The listing builds one solid part. Answer for the finished solid, in the listing's coordinates (mm). Face numbers are marked on the shaded views. A direction names the side the tool comes from. Coordinates: 2 decimals unless noted, no trailing zeros. Order: outer loops, then holes, each group sorted by start corner. A loop starts at its lowest first (then second) coordinate and runs counter-clockwise, first axis right, second up.
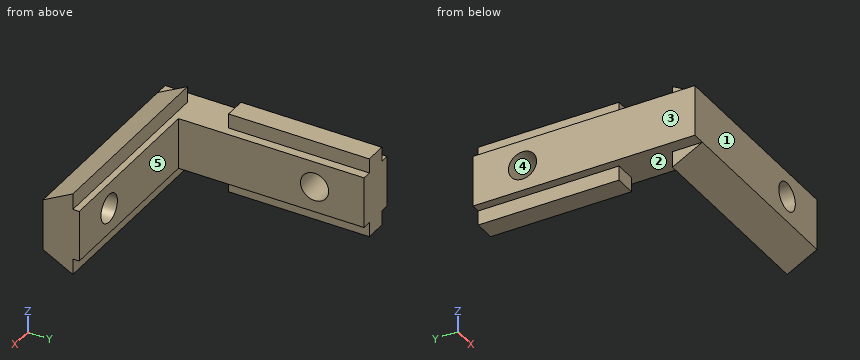
```python
from build123d import *

# Parameters (mm, degrees)
BOSS_EXTRUDE1_DEPTH   = 3
BOSS_EXTRUDE2_DEPTH   = 24
SKETCH3_W             = 1.3
SKETCH3_H             = 10.4
BOSS_EXTRUDE3_DEPTH   = 16.5
M4X0_7_TAPPED_HOLE1_D = 3.3
M4X0_7_TAPPED_HOLE2_D = 3.3
SKETCH9_W             = 3
SKETCH9_H             = 3
CUT_EXTRUDE1_DEPTH    = 38.329478968
MOVE_FACE1_BY         = 0.75
MOVE_FACE2_BY         = 0.4
MOVE_FACE3_BY         = 0.75
MOVE_FACE3_2_BY       = 0.75
MOVE_FACE4_BY         = 0.45
MOVE_FACE4_2_BY       = 0.45
MOVE_FACE5_BY         = 0.5
MOVE_FACE5_2_BY       = 0.5
MOVE_FACE6_BY         = 1
MOVE_FACE8_BY         = 0.25
MOVE_FACE8_2_BY       = 0.25


with BuildPart() as part:
    # Sketch1 → Boss-Extrude1 (new, symmetric)
    with BuildSketch(Plane.XY):
        with BuildLine():
            Line((0, 26), (0, 0))
            Line((0, 0), (25.5, 0))
            Line((25.5, 0), (25.5, 5))
            Line((25.5, 5), (8, 5))
            ThreePointArc((8, 5), (5.878679656, 5.878679656), (5, 8))
            Line((5, 8), (5, 26))
            Line((5, 26), (0, 26))
        make_face()
    extrude(amount=BOSS_EXTRUDE1_DEPTH, both=True)

    # Sketch2 → Boss-Extrude2 (add)
    with BuildSketch(Plane(origin=(25.5, 0, 0), x_dir=(0, 0, -1), z_dir=(1, 0, 0))):
        Polygon((-3, 0), (-5, 3.75), (5, 3.75), (3, 0), align=None)
    extrude(amount=-BOSS_EXTRUDE2_DEPTH)

    # Sketch3 → Boss-Extrude3 (add)
    with BuildSketch(Plane(origin=(0, 26, 0), x_dir=(1, 0, 0), z_dir=(0, 1, 0))):
        with Locations((2.15, 0)):
            Rectangle(SKETCH3_W, SKETCH3_H)
    extrude(amount=-BOSS_EXTRUDE3_DEPTH)

    # M4x0.7 Tapped Hole1 (through all)
    with Locations(Plane(origin=(0, 5, 0), x_dir=(1, 0, 0), z_dir=(0, 1, 0))):
        with Locations((18.5, 0)):
            Hole(M4X0_7_TAPPED_HOLE1_D / 2)

    # M4x0.7 Tapped Hole2 (through all)
    with Locations(Plane(origin=(5, 0, 0), x_dir=(0, 0, -1), z_dir=(1, 0, 0))):
        with Locations((0, 20.2)):
            Hole(M4X0_7_TAPPED_HOLE2_D / 2)

    # Sketch9 → Cut-Extrude1 (cut, through all)
    with BuildSketch(Plane(origin=(0, 0, -3), x_dir=(-1, 0, 0), z_dir=(0, 0, -1))):
        with Locations((-6.5, 6.5)):
            Rectangle(SKETCH9_W, SKETCH9_H)
    extrude(amount=-CUT_EXTRUDE1_DEPTH, mode=Mode.SUBTRACT)

    # Move Face1: a face moved inward by 0.75
    extrude(part.faces().sort_by_distance((15.007117259, 5, 0))[0], amount=MOVE_FACE1_BY, dir=(0, -1, 0), mode=Mode.SUBTRACT)

    # Move Face2: a face moved inward by 0.4
    extrude(part.faces().sort_by_distance((5, 14.769055213, 0))[0], amount=MOVE_FACE2_BY, dir=(-1, 0, 0), mode=Mode.SUBTRACT)

    # Move Face3: a face moved outward by 0.75
    extrude(part.faces().sort_by_distance((2.8, 17.75, 4.1))[0], amount=MOVE_FACE3_BY, dir=(1, 0, 0))

    # Move Face3 2: a face moved outward by 0.75
    extrude(part.faces().sort_by_distance((2.8, 17.75, -4.1))[0], amount=MOVE_FACE3_2_BY, dir=(1, 0, 0))

    # Move Face4: a face moved outward by 0.45
    extrude(part.faces().sort_by_distance((1.5, 17.75, 4.1))[0], amount=MOVE_FACE4_BY, dir=(-1, 0, 0))

    # Move Face4 2: a face moved outward by 0.45
    extrude(part.faces().sort_by_distance((1.5, 17.75, -4.1))[0], amount=MOVE_FACE4_2_BY, dir=(-1, 0, 0))

    # Move Face5: a face moved inward by 0.5
    extrude(part.faces().sort_by_distance((2.3, 17.75, 5.2))[0], amount=MOVE_FACE5_BY, dir=(0, 0, -1), mode=Mode.SUBTRACT)

    # Move Face5 2: a face moved inward by 0.5
    extrude(part.faces().sort_by_distance((2.3, 17.75, -5.2))[0], amount=MOVE_FACE5_2_BY, dir=(0, 0, 1), mode=Mode.SUBTRACT)

    # Move Face6: a face moved inward by 1.0
    extrude(part.faces().sort_by_distance((25.5, 2.210227273, 0))[0], amount=MOVE_FACE6_BY, dir=(-1, 0, 0), mode=Mode.SUBTRACT)

    # Move Face8: a face moved inward by 0.25
    extrude(part.faces().sort_by_distance((13, 3.75, -4))[0], amount=MOVE_FACE8_BY, dir=(0, -1, 0), mode=Mode.SUBTRACT)

    # Move Face8 2: a face moved inward by 0.25
    extrude(part.faces().sort_by_distance((13, 3.75, 4))[0], amount=MOVE_FACE8_2_BY, dir=(0, -1, 0), mode=Mode.SUBTRACT)


solid = part.part
```
(1) Consider line 1 (Y direction, x = 2, z = 0); line 2 (X direction, y = 9.5, z = 1); line 3 (Y direction, x = 21.5, z = 1). Determine where each line is inside the solid, lowest interval first.
(2) Each of these flat-tipped pins is pushed along its axis until it touches: pin 1 Ø1.4 at (y, z) = (18, -4) entering from +X; pin 2 Ø2 at (x, y) = (3, 21) entering from -Z; pin 3 Ø5.5 at (y, z) = (20.2, 0) entering from +X; pin 4 Ø5 at (y, z) = (11.5, -3.5) entering from -X. Where does it stop, or does it pass through?
(3) Find section A-A (y = 20.2). Write down the section's boundary in (x, z), and give its area (3 significant figures).
(4) Find section C-C (x = 21.75). Write down the section's boundary in (y, z).
(5) The mould has two halves that part along Y. Classify the marked faces 1, 2 and 3: released by +Y, released by -Y, zero draft, split by the parting line, or undercut.
(6) For the marked faces 4 and 5, determine the directions among +Z, -Z, +X, -X, +Y, -Y from which every point of the face is accessible in a straight line to the end or side of a thin tool.
(7) Find section B-B (z = -3.75). Write down the section's boundary in (x, y), and give its area (3 significant figures).
(8) Find section D-D (x = 18.5). Write down the section's boundary in (y, z), and give its area (3 significant figures).
Findings below:
1. line 1: y = 0 to 18.55, 21.85 to 26
1. line 2: x = 0 to 4.6
1. line 3: y = 0 to 4.25
2. pin 1: stops at x = 3.55
2. pin 2: stops at z = -4.7
2. pin 3: stops at x = 4.6
2. pin 4: stops at x = 0
3. outline: (0, -3) - (1.05, -3) - (1.05, -4.7) - (3.55, -4.7) - (3.55, -3) - (4.6, -3) - (4.6, -1.65) - (0, -1.65) - close; (0, 1.65) - (4.6, 1.65) - (4.6, 3) - (3.55, 3) - (3.55, 4.7) - (1.05, 4.7) - (1.05, 3) - (0, 3) - close
3. area: 20.9 mm2
4. outline: (0, -3) - (3.5, -4.87) - (3.5, -3) - (4.25, -3) - (4.25, 3) - (3.5, 3) - (3.5, 4.87) - (0, 3) - close
5. face 1: released by -Y
5. face 2: undercut
5. face 3: zero draft
6. face 4: +X, -X
6. face 5: +Z, -Z, +X, +Y
7. outline: (1.05, 9.5) - (3.55, 9.5) - (3.55, 26) - (1.05, 26) - close; (1.5, 1.41) - (24.5, 1.41) - (24.5, 3.5) - (1.5, 3.5) - close
7. area: 89.4 mm2
8. outline: (0, -3) - (3.5, -4.87) - (3.5, -3) - (4.25, -3) - (4.25, -1.65) - (0, -1.65) - close; (0, 1.65) - (4.25, 1.65) - (4.25, 3) - (3.5, 3) - (3.5, 4.87) - (0, 3) - close
8. area: 18.0 mm2
